Read the model definition and answer for the solid it produces. Units are mm, in the model's axes. Give positions to 0.01 mm unless a question says otherwise; leave off trailing zeros. Order: outer loops, then holes, each group sorted by start corner. A loop starts at its lowest first (then second) coordinate and runs counter-clockwise, first axis right, second up. Notation, with made-up numbers: (77, 6) - (121, 6) arc R32 ccw to (121, 38) - close; hole circle Ø11 at (11, 7.25). An arc over 180 degrees is marked (long way). Write each question's results on one line, items separated by ' | '. Start each with the question number.
Q1. Find section A-A on x = -82.5. Give the vertices of the cut face in (y, z), and give its area (3 significant figures).
Q2. Find the intervals of material crossed by line 1 along Z through (x, y) = (0, 1.7); line 2 along Z through (x, y) = (0, 298.5); line 3 along X through (y, z) = (31, 285.5), in increasing order. Write a range as from..to.
Q3. Find section D-D on y = 25.5. Give the vertices of the cut face in (x, z), and give its area (3 significant figures).
Q4. Find section C-C on y = 125. Give the vertices of the cut face in (x, z), and give its area (3 significant figures).
Q5. Flat-ended cylindrical pins translate along their axes: P1, Ø5, axis at y = 158.5, z = -118, coming from the +X side (3 decimals); P2, Ø4, axis at x = -257, y = 147, coming from the -Z side; P3, Ø1.5, axis at x = -112, y = 3.5, coming from the -Z side; P4, Ø10, axis at x = -170, y = 45.5, coming from the -Z side. Find the tip coordinate at first contact, or state that the pin passes through.
Q6. Find section B-B on z = 184. Give the vertices of the cut face in (x, y), and give its area (3 significant figures).
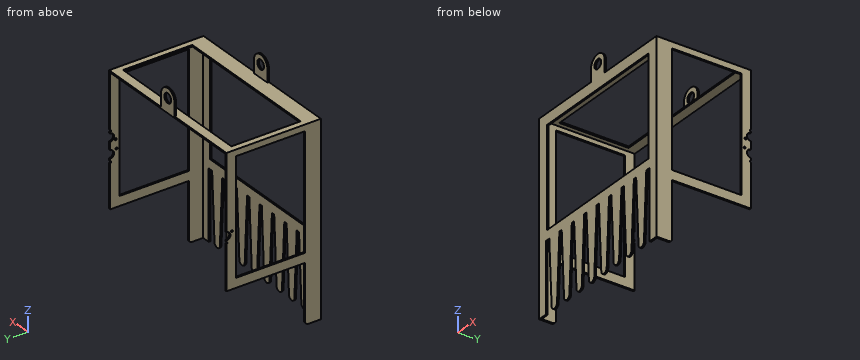
from build123d import *

# Parameters (mm, degrees)
EXTRUDE_1_DEPTH      = 300
SKETCH_2_W           = 480
SKETCH_2_H           = 220
CUT_EXTRUDE_1_DEPTH  = 601
SKETCH_3_W           = 364
SKETCH_3_H           = 220
CUT_EXTRUDE_2_DEPTH  = 520
SKETCH_5_W           = 186
SKETCH_5_H           = 250
CUT_EXTRUDE_4_DEPTH  = 520
SKETCH_6_W           = 510
SKETCH_6_H           = 800
CUT_EXTRUDE_5_DEPTH  = 295
CUT_EXTRUDE_3_REACH  = 522
SKETCH_4_R           = 12.5
SKETCH_12_R          = 12.5
CUT_EXTRUDE_8_DEPTH  = 10
SKETCH_7_R           = 15
EXTRUDE_2_DEPTH      = 300
CUT_EXTRUDE_6_REACH  = 292
SKETCH_8_W           = 177.621372849
SKETCH_8_H           = 290
SKETCH_10_W          = 450
SKETCH_10_H          = 315
CUT_EXTRUDE_7_DEPTH  = 51
FILLET_1_R           = 10
SKETCH_15_R          = 3
CUT_EXTRUDE_10_DEPTH = 5
SKETCH_16_R          = 3
CUT_EXTRUDE_11_DEPTH = 5
SKETCH_17_R          = 3
CUT_EXTRUDE_12_DEPTH = 5


with BuildPart() as part:
    # 草图1 → 凸台-拉伸1 (new body)
    with BuildSketch(Plane(origin=(0, 0, 0), x_dir=(1, 0, 0), z_dir=(0, 1, 0))):
        with BuildLine():
            Line((-215, 80), (-230, 80))
            Line((-230, 80), (-230, 300))
            Line((-230, 300), (-260, 300))
            Line((-260, 300), (-260, -300))
            Line((-260, -300), (260, -300))
            Line((260, -300), (260, 300))
            Line((260, 300), (230, 300))
            Line((230, 300), (230, 80))
            Line((230, 80), (215, 80))
            Line((215, 80), (204.484783483, 288.604123213))
            ThreePointArc((204.484783483, 288.604123213), (192.5, 300), (180.515216517, 288.604123213))
            Line((180.515216517, 288.604123213), (170, 80))
            Line((170, 80), (160, 80))
            Line((160, 80), (149.484783483, 288.604123213))
            ThreePointArc((149.484783483, 288.604123213), (137.5, 300), (125.515216517, 288.604123213))
            Line((125.515216517, 288.604123213), (115, 80))
            Line((115, 80), (105, 80))
            Line((105, 80), (94.484783483, 288.604123213))
            ThreePointArc((94.484783483, 288.604123213), (82.5, 300), (70.515216517, 288.604123213))
            Line((70.515216517, 288.604123213), (60, 80))
            Line((60, 80), (50, 80))
            Line((50, 80), (39.484783483, 288.604123213))
            ThreePointArc((39.484783483, 288.604123213), (27.5, 300), (15.515216517, 288.604123213))
            Line((15.515216517, 288.604123213), (5, 80))
            Line((5, 80), (-5, 80))
            Line((-5, 80), (-15.515216517, 288.604123213))
            ThreePointArc((-15.515216517, 288.604123213), (-27.5, 300), (-39.484783483, 288.604123213))
            Line((-39.484783483, 288.604123213), (-50, 80))
            Line((-50, 80), (-60, 80))
            Line((-60, 80), (-70.515216517, 288.604123213))
            ThreePointArc((-70.515216517, 288.604123213), (-82.5, 300), (-94.484783483, 288.604123213))
            Line((-94.484783483, 288.604123213), (-105, 80))
            Line((-105, 80), (-115, 80))
            Line((-115, 80), (-125.515216517, 288.604123213))
            ThreePointArc((-125.515216517, 288.604123213), (-137.5, 300), (-149.484783483, 288.604123213))
            Line((-149.484783483, 288.604123213), (-160, 80))
            Line((-160, 80), (-170, 80))
            Line((-170, 80), (-180.515216517, 288.604123213))
            ThreePointArc((-180.515216517, 288.604123213), (-192.5, 300), (-204.484783483, 288.604123213))
            Line((-204.484783483, 288.604123213), (-215, 80))
        make_face()
    extrude(amount=EXTRUDE_1_DEPTH)

    # 草图2 → 切除-拉伸1 (cut, through all)
    with BuildSketch(Plane.XY.offset(300)):
        with Locations((0, 160)):
            Rectangle(SKETCH_2_W, SKETCH_2_H)
    extrude(amount=-CUT_EXTRUDE_1_DEPTH, mode=Mode.SUBTRACT)

    # 草图3 → 切除-拉伸2 (cut)
    with BuildSketch(Plane.ZY.offset(260)):
        with Locations((98, 160)):
            Rectangle(SKETCH_3_W, SKETCH_3_H)
    extrude(amount=-CUT_EXTRUDE_2_DEPTH, mode=Mode.SUBTRACT)

    # 草图5 → 切除-拉伸4 (cut)
    with BuildSketch(Plane.ZY.offset(260)):
        with Locations((-207, 175)):
            Rectangle(SKETCH_5_W, SKETCH_5_H)
    extrude(amount=-CUT_EXTRUDE_4_DEPTH, mode=Mode.SUBTRACT)

    # 草图6 → 切除-拉伸5 (cut)
    with BuildSketch(Plane(origin=(0, 300, 0), x_dir=(1, 0, 0), z_dir=(0, 1, 0))):
        with Locations((0, 105)):
            Rectangle(SKETCH_6_W, SKETCH_6_H)
    extrude(amount=-CUT_EXTRUDE_5_DEPTH, mode=Mode.SUBTRACT)

    # 草图4 → 切除-拉伸3 (cut, up to next)
    with BuildSketch(Plane.ZY.offset(260), mode=Mode.PRIVATE) as cut_extrude_3_sk1:
        with Locations((50, 300)):
            Circle(SKETCH_4_R)
    cut_extrude_3_tool1 = extrude(cut_extrude_3_sk1.sketch, amount=-CUT_EXTRUDE_3_REACH, mode=Mode.PRIVATE) & part.part
    add(cut_extrude_3_tool1.solids().sort_by_distance((-260, 300, 50))[0], mode=Mode.SUBTRACT)

    # 草图12 → 切除-拉伸8 (cut)
    with BuildSketch(Plane(origin=(260, 0, 0), x_dir=(0, 0, -1), z_dir=(1, 0, 0))):
        with Locations((-100, 300)):
            Circle(SKETCH_12_R)
        with Locations((-50, 300)):
            Circle(SKETCH_12_R)
    extrude(amount=-CUT_EXTRUDE_8_DEPTH, mode=Mode.SUBTRACT)

    # 草图7 → 凸台-拉伸2 (add)
    with BuildSketch(Plane(origin=(0, 300, 0), x_dir=(1, 0, 0), z_dir=(0, 1, 0))):
        with BuildLine():
            Line((-30, -340), (-30, -300))
            Line((-30, -300), (30, -300))
            Line((30, -300), (30, -340))
            ThreePointArc((30, -340), (0, -370), (-30, -340))
        make_face()
        with Locations((0, -340)):
            Circle(SKETCH_7_R, mode=Mode.SUBTRACT)
    extrude(amount=-EXTRUDE_2_DEPTH)

    # 草图8 → 切除-拉伸6 (cut, up to next)
    with BuildSketch(Plane.ZY.offset(30), mode=Mode.PRIVATE) as cut_extrude_6_sk1:
        with Locations((388.810686424, 150)):
            Rectangle(SKETCH_8_W, SKETCH_8_H)
    cut_extrude_6_tool1 = extrude(cut_extrude_6_sk1.sketch, amount=-CUT_EXTRUDE_6_REACH, mode=Mode.PRIVATE) & part.part
    add(cut_extrude_6_tool1.solids().sort_by_distance((-30, 150, 388.810686))[0], mode=Mode.SUBTRACT)

    # 草图10 → 切除-拉伸7 (cut, through all)
    with BuildSketch(Plane(origin=(0, 50, 0), x_dir=(1, 0, 0), z_dir=(0, 1, 0))):
        with Locations((0, -107.5)):
            Rectangle(SKETCH_10_W, SKETCH_10_H)
    extrude(amount=-CUT_EXTRUDE_7_DEPTH, mode=Mode.SUBTRACT)

    # 圆角1
    fillet_1_edges = [part.edges().sort_by_distance(p)[0] for p in [
        (-257.5, 50, -300),
        (257.5, 50, -300),
    ]]
    fillet(fillet_1_edges, radius=FILLET_1_R)

    # 草图15 → 切除-拉伸10 (cut)
    with BuildSketch(Plane(origin=(260, 0, 0), x_dir=(0, 0, -1), z_dir=(1, 0, 0))):
        with Locations((-120, 300)):
            Circle(SKETCH_15_R)
        with Locations((-90, 282.679491924)):
            Circle(SKETCH_15_R)
    extrude(amount=-CUT_EXTRUDE_10_DEPTH, mode=Mode.SUBTRACT)

    # 草图16 → 切除-拉伸11 (cut)
    with BuildSketch(Plane.ZY.offset(260)):
        with Locations((30, 300)):
            Circle(SKETCH_16_R)
        with Locations((60, 282.679491924)):
            Circle(SKETCH_16_R)
    extrude(amount=-CUT_EXTRUDE_11_DEPTH, mode=Mode.SUBTRACT)

    # 草图17 → 切除-拉伸12 (cut)
    with BuildSketch(Plane(origin=(260, 0, 0), x_dir=(0, 0, -1), z_dir=(1, 0, 0))):
        with Locations((-27, 300)):
            Circle(SKETCH_17_R)
        with Locations((-61.5, 280.081415713)):
            Circle(SKETCH_17_R)
    extrude(amount=-CUT_EXTRUDE_12_DEPTH, mode=Mode.SUBTRACT)


solid = part.part
Working result:
1) outline: (0, -300) - (5, -300) - (5, -50) - (0, -50) - close; (0, 265) - (5, 265) - (5, 295) - (50, 295) - (50, 300) - (0, 300) - close; (270, 295) - (300, 295) - (300, 300) - (270, 300) - close | area: 1,800 mm²
2) line 1: -80..-50, 265..325, 355..370 | line 2: 295..325, 355..370 | line 3: -260..-255, 255..260
3) outline: (-260, -300) - (-255, -300) - (-255, 295) - (255, 295) - (255, -300) - (260, -300) - (260, 300) - (-260, 300) - close | area: 8,550 mm²
4) outline: (-260, -114) - (-255, -114) - (-255, -84) - (-260, -84) - close; (-260, 280) - (-255, 280) - (-255, 295) - (-240, 295) - (-240, 300) - (-260, 300) - close; (240, 295) - (255, 295) - (255, 280) - (260, 280) - (260, 300) - (240, 300) - close; (255, -114) - (260, -114) - (260, -84) - (255, -84) - close | area: 650 mm²
5) P1: through | P2: z = -114 | P3: z = -80 | P4: z = 295
6) outline: (-260, 0) - (-225, 0) - (-225, 5) - (-255, 5) - (-255, 50) - (-260, 50) - close; (-260, 270) - (-255, 270) - (-255, 300) - (-260, 300) - close; (225, 0) - (260, 0) - (260, 50) - (255, 50) - (255, 5) - (225, 5) - close; (255, 270) - (260, 270) - (260, 300) - (255, 300) - close | area: 1,100 mm²
